from build123d import *

# Parameters (mm, degrees)
F0_W     = 22
F0_H     = 3
F1_DEPTH = 142.5
F3_D     = 4.3
F3_DEPTH = 3
F3_TIP   = 1.2918503309
F5_D     = 4
F5_DEPTH = 3
F5_TIP   = 1.2017212381
F7_DEPTH = 100


with BuildPart() as f1:
    # F0 (on Front) → F1 (new body, symmetric)
    with BuildSketch(Plane.XZ):
        with Locations((12.5, 48.5)):
            Rectangle(F0_W, F0_H)
        Polygon((1.5, 47), (1.5, 50), (-1.5, 50), (-1.5, -50), (1.5, -50), align=None)
    extrude(amount=F1_DEPTH, both=True)

    # F3
    with Locations(Plane(origin=(-1.5, 0, 0), x_dir=(0, -1, 0), z_dir=(-1, 0, 0))):
        with Locations((-92.5, 43), (-66.5, 43), (66.5, 43), (92.5, 43)):
            Hole(F3_D / 2, depth=F3_DEPTH)
            with Locations((0, 0, -(F3_DEPTH + F3_TIP / 2))):  # 118° drill point
                Cone(0, F3_D / 2, F3_TIP, mode=Mode.SUBTRACT)

    # F5
    with Locations(Plane.XY.offset(50)):
        with Locations((10.5, 92.5), (10.5, 0), (10.5, -92.5)):
            Hole(F5_D / 2, depth=F5_DEPTH)
            with Locations((0, 0, -(F5_DEPTH + F5_TIP / 2))):  # 118° drill point
                Cone(0, F5_D / 2, F5_TIP, mode=Mode.SUBTRACT)

    # F6 (on face) → F7 (cut)
    with BuildSketch(Plane.XY.offset(50)):
        Polygon((23.5, 142.5), (-1.5, 142.5), (23.5, 117.5), align=None)
        Polygon((23.5, -117.5), (-1.5, -142.5), (23.5, -142.5), align=None)
    extrude(amount=-F7_DEPTH, mode=Mode.SUBTRACT)


solid = f1.part
Read the model definition and answer for the solid it produces. Units are mm, in the model's axes. A direction names the side the tool comes from. Round coordinates to 2 decimals unless told otherwise and drop trailing zeros. Write each loop counter-clockwise with the first axis right and the second up, starting at its lowest first coordinate (ties: lowest second). Pieces come first, ordered by that corner, then holes.
Q1. Find section C-C on z = -29. Determine the outline of the cut face in (x, y), and give its area (3 significant figures).
Values:
outline: (-1.5, -142.5) - (1.5, -139.5) - (1.5, 139.5) - (-1.5, 142.5) - close
area: 846 mm2
Q2. Flat-ended cylindrical pins translate along their axes: P1, Ø6, axis at y = 106.5, z = 16.5, coming from the +X side; P2, Ø7, axis at y = 92.5, z = 43, coming from the -X side; P3, Ø5, axis at x = 10.5, y = -92.5, coming from the -Z side; P4, Ø3, axis at x = 10.5, y = 92.5, coming from the +Z side. Find the tip coordinate at first contact, or state that the pin passes through.
Values:
P1: stops at x = 1.5
P2: stops at x = -1.5
P3: stops at z = 47
P4: passes through
Q3. Find section B-B on x = 5. Determine the outline of the cut face in (y, z).
Values:
outline: (-136, 47) - (136, 47) - (136, 50) - (-136, 50) - close
Q4. Find section A-A on y = -25. Determine the outline of the cut face in (x, z), and give its area (3 significant figures).
Values:
outline: (-1.5, -50) - (1.5, -50) - (1.5, 47) - (23.5, 47) - (23.5, 50) - (-1.5, 50) - close
area: 366 mm2
Q5. Straight lines are drawn through the part: line 1 (X direction, y = 0, z = 48); line 2 (Y direction, x = 10.5, z = 48.55); line 3 (X direction, y = 24, z = 40). For each, find the intervals that lie inside material, in ascending order.
Values:
line 1: x = -1.5 to 8.5, 12.5 to 23.5
line 2: y = -130.5 to -94.5, -90.5 to -2, 2 to 90.5, 94.5 to 130.5
line 3: x = -1.5 to 1.5
Q6. A tool of negligible diameter and unlimited length cuts with its end or side. For faces 1 (the face through (1, 140, 11)), 2 (the face through (1.5, -2, -2)), from which of +Z, -Z, +X, -X, +Y, -Y can it reach the whole face along a straight path? Write none if from no direction.
Values:
face 1: +Z, -Z, +X, +Y
face 2: -Z, +X, +Y, -Y
